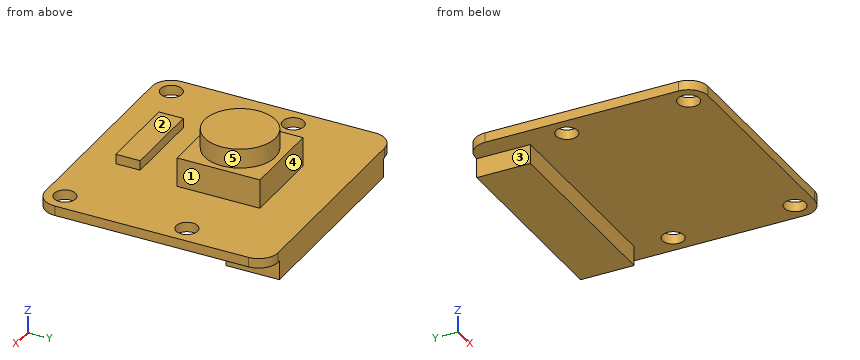
```python
from build123d import *

# Parameters (mm, degrees)
SKETCH1_W           = 25
SKETCH1_H           = 23.862
BOSS_EXTRUDE1_DEPTH = 1
FILLET1_R           = 2
SKETCH2_R           = 1.1
CUT_EXTRUDE1_DEPTH  = 1
SKETCH3_W           = 8.5
SKETCH3_H           = 2.5
SKETCH3_H_2         = 8.5
BOSS_EXTRUDE2_DEPTH = 1
SKETCH4_W           = 8.5
SKETCH4_H           = 8.5
BOSS_EXTRUDE3_DEPTH = 2
SKETCH5_R           = 3.625
BOSS_EXTRUDE4_DEPTH = 2
SKETCH6_W           = 20.5
SKETCH6_H           = 5.5
BOSS_EXTRUDE5_DEPTH = 2


with BuildPart() as part:
    # Sketch1 → Boss-Extrude1 (new body)
    with BuildSketch(Plane.XY):
        Rectangle(SKETCH1_W, SKETCH1_H)
    extrude(amount=BOSS_EXTRUDE1_DEPTH)

    # Fillet1
    fillet1_edges = [part.edges().sort_by_distance(p)[0] for p in [
        (12.5, -11.931, 0.5),
        (-12.5, -11.931, 0.5),
        (-12.5, 11.931, 0.5),
        (12.5, 11.931, 0.5),
    ]]
    fillet(fillet1_edges, radius=FILLET1_R)

    # Sketch2 → Cut-Extrude1 (cut)
    with BuildSketch(Plane.XY.offset(1)):
        with Locations((-10.5, -9.931)):
            Circle(SKETCH2_R)
        with Locations((10.5, -9.931)):
            Circle(SKETCH2_R)
        with Locations((10.5, 2.569)):
            Circle(SKETCH2_R)
        with Locations((-10.5, 2.569)):
            Circle(SKETCH2_R)
    extrude(amount=-CUT_EXTRUDE1_DEPTH, mode=Mode.SUBTRACT)

    # Sketch3 → Boss-Extrude2 (add)
    with BuildSketch(Plane.XY.offset(1)):
        with Locations((-1, -7.231)):
            Rectangle(SKETCH3_W, SKETCH3_H)
        with Locations((0, 2.569)):
            Rectangle(SKETCH3_W, SKETCH3_H_2)
    extrude(amount=BOSS_EXTRUDE2_DEPTH)

    # Sketch4 → Boss-Extrude3 (add)
    with BuildSketch(Plane.XY.offset(2)):
        with Locations((0, 2.569)):
            Rectangle(SKETCH4_W, SKETCH4_H)
    extrude(amount=BOSS_EXTRUDE3_DEPTH)

    # Sketch5 → Boss-Extrude4 (add)
    with BuildSketch(Plane.XY.offset(4)):
        with Locations((0, 2.569)):
            Circle(SKETCH5_R)
    extrude(amount=BOSS_EXTRUDE4_DEPTH)

    # Sketch6 → Boss-Extrude5 (add)
    with BuildSketch(Plane(origin=(0, 0, 0), x_dir=(-1, 0, 0), z_dir=(0, 0, -1))):
        with Locations((0, 9.181)):
            Rectangle(SKETCH6_W, SKETCH6_H)
    extrude(amount=BOSS_EXTRUDE5_DEPTH)


solid = part.part
```
Verification items for the finished model (mm, model axes). Face numbers are marked on the shaded views. A direction names the side the tool comes from. Coordinates: 2 decimals unless noted, no trailing zeros. Order: outer loops, then holes, each group sorted by start corner. A loop starts at its lowest first (then second) coordinate and runs counter-clockwise, first axis right, second up. Notation, with made-up numbers: (-6, -30) -> (27, -30) arc R16 ccw to (27, -13) -> close; hole circle Ø7 at (70, 40.5). An arc over 180 degrees is marked (long way). Answer as CSV lines item,"result". Start each with the question number.
1) Set-up check for the marked faces 1, 2, 3, 4 and 5: record each of +Z, -Z, +X, -X, +Y, -Y from which the full face is reachable in a straight line by a thin tool's end or side.
2) Material ranges on L1, parallel to Y at x = -10.5, z = 0.5; L2, parallel to Z at x = 6, y = 10.5; L3, parallel to Y at x = -1.25, z = 1.25, recorded low to high. Write a range as [from, to].
3) Gauge pin test, flat ends, axial feed: pin 1 Ø3.5 at (x, y) = (10.5, 2.569) entering from +Z; pin 2 Ø2 at (x, y) = (-0.5, -7.5) entering from +Z; pin 3 Ø2.5 at (y, z) = (1, 2.5) entering from -X; pin 4 Ø2 at (x, z) = (-10, 3.5) entering from +Y (3 decimals). Record the tip position at first contact, or that the pin passes through.
4) Cross-section at B-B, the plane x = 0. Record the boundary of the cut face in (y, z).
5) Cross-section at C-C, the plane y = 7.25. Record the boundary of the cut face in (x, z), then the cut area to 3 significant figures.
6) Cross-section at A-A, the plane z = 1.5. Record the boundary of the cut face in (x, y).
7) Cross-section at D-D, the plane x = 2.5. Record the boundary of the cut face in (y, z).
Conclusion:
1,face 1,"+Z, +X, +Y, -Y"
1,face 2,"+Z, +X, -X, -Y"
1,face 3,"-Z, -X, +Y, -Y"
1,face 4,"+Z, +X, -X, +Y"
1,face 5,"+Z"
2,L1,"y = [-11.93, -11.03], [-8.83, 1.47], [3.67, 11.93]"
2,L2,"z = [-2, 1]"
2,L3,"y = [-8.48, -5.98], [-1.68, 6.82]"
3,pin 1,"stops at z = 1"
3,pin 2,"stops at z = 2"
3,pin 3,"stops at x = -4.25"
3,pin 4,"passes through"
4,outline,"(-11.93, 0) -> (6.43, 0) -> (6.43, -2) -> (11.93, -2) -> (11.93, 1) -> (6.82, 1) -> (6.82, 4) -> (6.19, 4) -> (6.19, 6) -> (-1.06, 6) -> (-1.06, 4) -> (-1.68, 4) -> (-1.68, 1) -> (-5.98, 1) -> (-5.98, 2) -> (-8.48, 2) -> (-8.48, 1) -> (-11.93, 1) -> close"
5,outline,"(-12.5, 0) -> (-10.25, 0) -> (-10.25, -2) -> (10.25, -2) -> (10.25, 0) -> (12.5, 0) -> (12.5, 1) -> (-12.5, 1) -> close"
5,area,"66.0 mm²"
6,outline,"(-5.25, -8.48) -> (3.25, -8.48) -> (3.25, -5.98) -> (-5.25, -5.98) -> close; (-4.25, -1.68) -> (4.25, -1.68) -> (4.25, 6.82) -> (-4.25, 6.82) -> close"
7,outline,"(-11.93, 0) -> (6.43, 0) -> (6.43, -2) -> (11.93, -2) -> (11.93, 1) -> (6.82, 1) -> (6.82, 4) -> (5.19, 4) -> (5.19, 6) -> (-0.06, 6) -> (-0.06, 4) -> (-1.68, 4) -> (-1.68, 1) -> (-5.98, 1) -> (-5.98, 2) -> (-8.48, 2) -> (-8.48, 1) -> (-11.93, 1) -> close"
